Print and shaded views of the part. All mm, measured from the part's lowest x, y and z. Round coordinates to 2 decimals unless told otherwise and drop trailing zeros. Write each loop counter-clockwise with the first axis right and the second up, starting at its lowest first coordinate (ties: lowest second). Pieces come first, ordered by that corner, then holes. Notation, with made-up numbers: M 20,89.5 L 69,89.5 A19 ccw 69,124.5 Z; hole C -16,-36.5 d8. An arc over 180 degrees is marked long. Write item = value, one per line. Start each with the question number.
Q1. Drop a flat-ended pin along its axis: P1, Ø2.5, axis at x = 127, z = 120.65, coming from the -Y side. Give the stop position or say it passes through.
Q2. Band-saw the part on C-C on z = 24.13. Write the cut outline in (x, y) (1 decimal), plus the area to 3 significant figures.
Q3. Band-saw the part on A-A on x = 25.4. Write the cut outline in (y, z) (1 decimal), plus the area to 3 significant figures.
Q4. Probe L1, parallel to X at y = 6.5, z = 24.13; L2, parallel to X at y = 3.5, z = 120.65; L3, parallel to Z at x = 148.59, y = 5.5. List the from-to ranges inside material, lowest first.
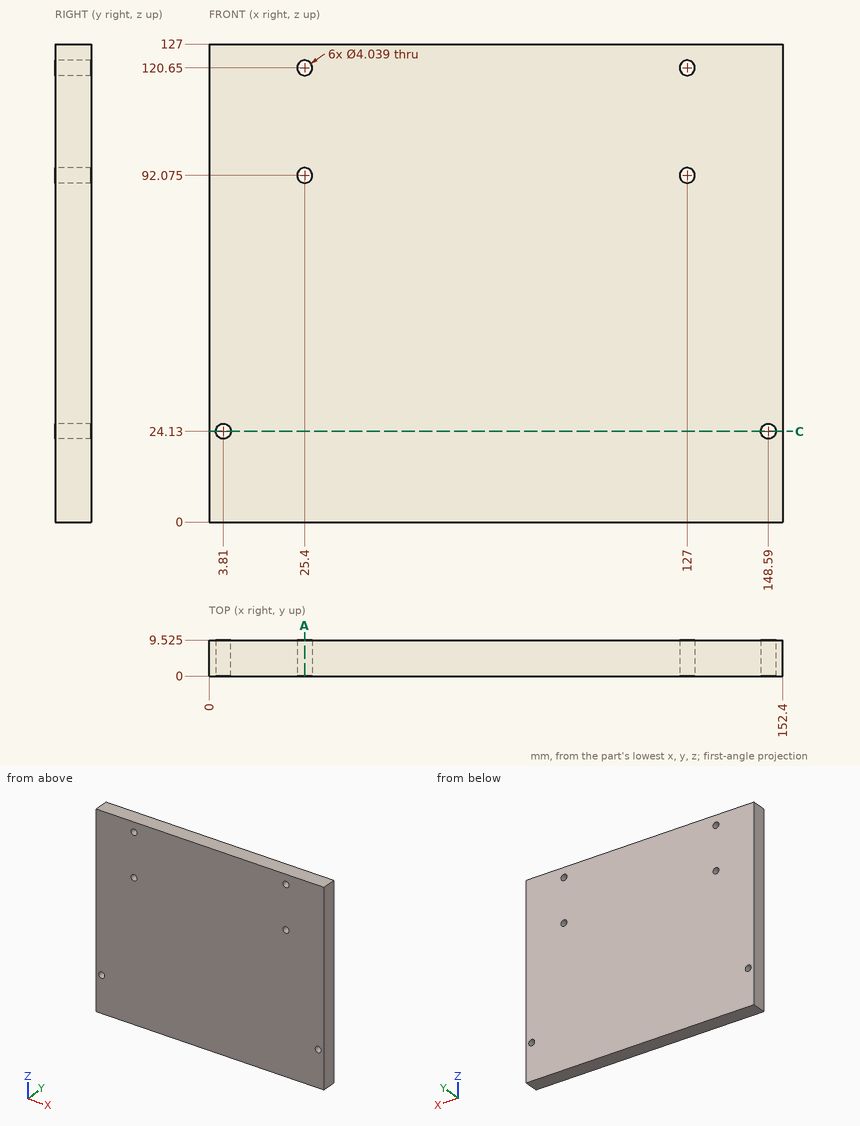
Conclusion:
q1.P1 = through
q2.outline = M 0,0 L 1.8,0 L 1.8,9.5 L 0,9.5 Z; M 5.8,0 L 146.6,0 L 146.6,9.5 L 5.8,9.5 Z; M 150.6,0 L 152.4,0 L 152.4,9.5 L 150.6,9.5 Z
q2.area = 1,370 mm^2
q3.outline = M 0,0 L 9.5,0 L 9.5,90.1 L 0,90.1 Z; M 0,94.1 L 9.5,94.1 L 9.5,118.6 L 0,118.6 Z; M 0,122.7 L 9.5,122.7 L 9.5,127 L 0,127 Z
q3.area = 1,130 mm^2
q4.L1 = 0 to 1.79, 5.83 to 146.57, 150.61 to 152.4
q4.L2 = 0 to 23.38, 27.42 to 124.98, 129.02 to 152.4
q4.L3 = 0 to 22.11, 26.15 to 127
